Verification items for the finished model (mm, model axes). Give positions to 0.01 mm unless a question says otherwise; leave off trailing zeros. Loops run counter-clockwise (first coordinate to the right, second up) from the corner with the lowest first, then second, coordinate; pieces in that order, holes last. Notation, with made-up numbers: (-17.5, 69) - (23.5, 69) arc R25 ccw to (23.5, 86) - close; hole circle Ø6 at (-35.5, 22). An arc over 180 degrees is marked (long way). Use one line per item in the form item = value.
```python
from build123d import *

# Parameters (mm, degrees)
PAD_DEPTH       = 300
SKETCH001_R     = 3
POCKET_DEPTH    = 17.410023
SKETCH002_R     = 5
POCKET001_DEPTH = 5


with BuildPart() as part:
    # Sketch → Pad (new body)
    with BuildSketch(Plane.XY):
        with BuildLine():
            Line((-9.5, 0), (9.5, 0))
            ThreePointArc((9.5, 0), (9.928584, 0.242481), (9.941474, 0.734736))
            Line((4, 11.909023), (9.941474, 0.734736))
            Line((9.810688, 16.517266), (4, 11.909023))
            ThreePointArc((9.810688, 16.517266), (9.972164, 17.073525), (9.5, 17.409023))
            Line((9.5, 17.409023), (-9.5, 17.409023))
            ThreePointArc((-9.5, 17.409023), (-9.972164, 17.073525), (-9.810688, 16.517266))
            Line((-9.810688, 16.517266), (-4, 11.909023))
            Line((-4, 11.909023), (-9.941474, 0.734736))
            ThreePointArc((-9.941474, 0.734736), (-9.928584, 0.242481), (-9.5, 0))
        make_face()
    extrude(amount=PAD_DEPTH)

    # Sketch001 (on Face2 of Pad) → Pocket (cut, through all)
    with BuildSketch(Plane(origin=(0, 17.409023, 0), x_dir=(-1, 0, 0), z_dir=(0, 1, 0))):
        with Locations((0, 20)):
            Circle(SKETCH001_R)
        with Locations((0, 80)):
            Circle(SKETCH001_R)
        with Locations((0, 140)):
            Circle(SKETCH001_R)
        with Locations((0, 200)):
            Circle(SKETCH001_R)
        with Locations((0, 260)):
            Circle(SKETCH001_R)
    extrude(amount=-POCKET_DEPTH, mode=Mode.SUBTRACT)

    # Sketch002 (on Face3 of Pocket) → Pocket001 (cut)
    with BuildSketch(Plane(origin=(0, 17.409023, 0), x_dir=(-1, 0, 0), z_dir=(0, 1, 0))):
        with Locations((0, 260)):
            Circle(SKETCH002_R)
        with Locations((0, 200)):
            Circle(SKETCH002_R)
        with Locations((0, 140)):
            Circle(SKETCH002_R)
        with Locations((0, 80)):
            Circle(SKETCH002_R)
        with Locations((0, 20)):
            Circle(SKETCH002_R)
    extrude(amount=-POCKET001_DEPTH, mode=Mode.SUBTRACT)


solid = part.part
```
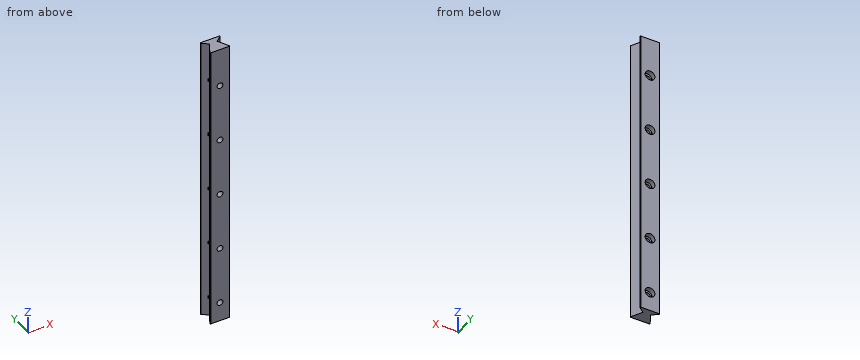
1. Section check B-B, the plane x = 0. State how many separate pieces and enclosed holes the cut face has, then the cut area to 3 significant figures.
Result set:
separate_pieces = 6
enclosed_holes = 0
area = 4,600 mm²
2. Scan lines: probe 1 along Z at (x, y) = (0, 16.2); probe 2 along Z at (x, y) = (0, 5); probe 3 along Y at (x, z) = (-9, 275.5). Record each from-to range of solid material in increasing order.
Result set:
probe_1 = 0 to 15, 25 to 75, 85 to 135, 145 to 195, 205 to 255, 265 to 300
probe_2 = 0 to 17, 23 to 77, 83 to 137, 143 to 197, 203 to 257, 263 to 300
probe_3 = 0 to 2.51, 15.87 to 17.41
3. Section check A-A, the plane z = 49. Record the cut outline in (x, y), then the cut area to 3 significant figures.
Result set:
outline = (-9.94, 0.73) arc R0.5 ccw to (-9.5, 0) - (9.5, 0) arc R0.5 ccw to (9.94, 0.73) - (4, 11.91) - (9.81, 16.52) arc R0.5 ccw to (9.5, 17.41) - (-9.5, 17.41) arc R0.5 ccw to (-9.81, 16.52) - (-4, 11.91) - close
area = 252 mm²
4. Depth check by flat-ended pin: pin 1 Ø4.5 at (x, z) = (-0.5, 261) entering from +Y; pin 2 Ø11.5 at (x, z) = (0, 20) entering from -Y. Enter the tip coordinate at first touch or a pass-through.
Result set:
pin_1 = 12.41
pin_2 = 0
